Could you check a few things on this model? Use its own coordinates, in mm. A direction names the side the tool comes from. Round coordinates to 2 decimals unless told otherwise and drop trailing zeros. Write each loop counter-clockwise with the first axis right and the second up, starting at its lowest first coordinate (ties: lowest second). Pieces come first, ordered by that corner, then holes. Notation, with made-up numbers: (36, 26) - (76, 26) arc R24 ccw to (76, 61) - close; hole circle Ø8 at (16.25, -10.75). An arc over 180 degrees is marked (long way). Put each result on its own line as item: value.
Autodesk Inventor part; units mm, degrees
ref_plane "YZ Plane" through (0, 0, 0) normal (1, 0, 0) x (0, 1, 0)
ref_plane "XZ Plane" through (0, 0, 0) normal (0, 1, 0) x (-1, 0, 0)
ref_plane "XY Plane" through (0, 0, 0) normal (0, 0, 1) x (1, 0, 0)
sketch "スケッチ1" plane through (0, 0, 0) normal (0, 0, 1) x (1, 0, 0)
  circle A0 centre (0, 0) radius 27.25
  line L0 (17.5, 17.5) -> (-17.5, 17.5)
  line L1 (-17.5, 17.5) -> (-17.5, -17.5)
  line L2 (-17.5, -17.5) -> (17.5, -17.5)
  line L3 (17.5, -17.5) -> (17.5, 17.5)
  line L4 (17.5, 17.5) -> (-17.5, -17.5) construction
  line L5 (-17.5, 17.5) -> (17.5, -17.5) construction
  line L6 (1, 17.5) -> (-1, 17.5)
  line L7 (-1, 17.5) -> (-1, -17.5)
  line L8 (-1, -17.5) -> (1, -17.5)
  line L9 (1, -17.5) -> (1, 17.5)
  line L10 (1, 17.5) -> (-1, -17.5) construction
  line L11 (-1, 17.5) -> (1, -17.5) construction
  point P0 (1, -17.5)
  point P1 (1, 17.5)
  point P2 (-1, 17.5)
  point P3 (-1, -17.5)
  dimension "d0" = 54.5
  dimension "d6" = 35
  dimension "d107" = 2
  dimension "d108" = 35
extrude "押し出し1" add sketch "スケッチ1" against normal blind 3 contours A0 | L9 L2 L7 L0
sketch "スケッチ2" plane through (0, 0, 0) normal (0, 0, 1) x (1, 0, 0)
  line L0 (0, 42.4511) -> (0, -37.5489)
  line L1 (38.0038, 0) -> (-41.9962, 0)
  line L2 (27.25, 42.0143) -> (27.25, -37.9857)
  circle A0 centre (0, 0) radius 27.25
  line L3 (17.5, 17.5) -> (17.5, -17.5)
  line L4 (19.25, 25) -> (27.25, 25)
  line L5 (27.25, 25) -> (27.25, -25)
  line L6 (27.25, -25) -> (19.25, -25)
  line L7 (19.25, -25) -> (19.25, 25)
  line L8 (19.25, 25) -> (27.25, -25) construction
  line L9 (27.25, 25) -> (19.25, -25) construction
  point P0 (17.5, 0)
  point P1 (23.25, 0)
  point P2 (19.25, 0)
  point P3 (27.25, 0)
  dimension "d13" = 9.75
  dimension "d14" = 8
  dimension "d15" = 50
  dimension "d19" = 54.5
  dimension "d110" = 1.75
extrude "押し出し2" cut sketch "スケッチ2" against normal blind 10 contours L7 L4 L2 A0 | A0 L1 L7 picked at (20.3822, 11.481)
mirror "ミラー1" about plane through (0, 0, 0) normal (1, 0, 0) of "押し出し2"
sketch "スケッチ8" plane through (0, 0, 0) normal (0, 0, 1) x (1, 0, 0)
  circle A0 centre (0, 0) radius 22.375
  circle A1 centre (0, 0) radius 27.25
  line L0 (0, 31.1603) -> (0, -30.8706)
  point P0 (0, 0)
  point P1 (0, 22.375)
  point P2 (0, -22.375)
  dimension "d112" = 44.75
  dimension "d113" = 54.5
hole "穴5" at (0, 22.375, 0) at (0, -22.375, 0) direction (0, 0, -1) diameter 4.5 end through all
properties part number "Part3_A_Y" material "鋼、軟鋼"
(1) If we mould it in two halves opening along Y, with no side actions, what happens to faces 6 (the face through (0.3, 27.25, -1.48)), 7 (the face through (-9, 17.5, -1)), 8 (the face through (0, 0, -3))? For each: pulls with the +Y half, pulls with the -Y half, needs draft (parallel to the pull), parting line crosses it, or undercut.
Values found:
face 6: pulls with the +Y half
face 7: undercut
face 8: needs draft
(2) I'm going to push flat-ended pins straight in: pin 1 (1 mm diameter, centred on y = 11.5, z = -0.5, fed in from +X); pin 2 (2.5 mm diameter, centred on x = 0, y = -22.375, fed in from -Z); pin 3 (0.9 mm diameter, centred on y = 2.5, z = -1, fed in from -X); pin 4 (0.9 mm diameter, centred on x = 10, z = -2, fed in from +Y). Where does each tip first touch, or does it pass through?
Values found:
pin 1: stops at x = 19.25
pin 2: passes through
pin 3: stops at x = -19.25
pin 4: stops at y = 25.52
(3) Imagine slicing it at D-D, the plane x = -23.5. List the corners of the cut face in (y, z) for me.
Values found:
outline: (-13.8, -3) - (0, -3) - (0, 0) - (-13.8, 0) - close
(4) For faces 1 (the face through (-23, 0, -1)), 2 (the face through (-0.599, -27.243, -1.479)), 3 (the face through (0, 0, 0)), 4 (the face through (9, 17.5, -1)), 5 (the face through (19.25, 10, -1)), which set-ups out of +Z, -Z, +X, -X, +Y, -Y let a thin tool reach every point of the face, with its end or its side?
Values found:
face 1: +Z, -Z, -X, +Y
face 2: +Z, -Z, -Y
face 3: +Z, +X, -X, +Y, -Y
face 4: +Z, -Z
face 5: +Z, -Z, +X, +Y
(5) Imagine slicing it at A-A, the plane x = 0. List the corners of the cut face in (y, z) for me (3 decimals).
Values found:
outline: (-27.25, -3) - (-24.625, -3) - (-24.625, 0) - (-27.25, 0) - close; (-20.125, -3) - (20.125, -3) - (20.125, 0) - (-20.125, 0) - close; (24.625, -3) - (27.25, -3) - (27.25, 0) - (24.625, 0) - close
(6) Imagine slicing it at B-B, the plane y = 14. List the corners of the cut face in (x, z) for me.
Values found:
outline: (-19.25, -3) - (-17.5, -3) - (-17.5, 0) - (-19.25, 0) - close; (-1, -3) - (1, -3) - (1, 0) - (-1, 0) - close; (17.5, -3) - (19.25, -3) - (19.25, 0) - (17.5, 0) - close
(7) Please list where these lines run through material, in increasing order: probe 1 along Y at (x, z) = (0, -0.9) (3 decimals); probe 2 along X at (y, z) = (12, -2.6); probe 3 along X at (y, z) = (-7, -2.45). Write a range as from..to.
Values found:
probe 1: y = -27.25..-24.625, -20.125..20.125, 24.625..27.25
probe 2: x = -19.25..-17.5, -1..1, 17.5..19.25
probe 3: x = -26.34..-17.5, -1..1, 17.5..26.34
(8) Imagine slicing it at C-C, the plane z = -0.55. List the corners of the cut face in (x, y) for me (3 decimals), then the cut area to 3 significant figures.
Values found:
outline: (-27.25, 0) arc R27.25 ccw to (27.25, 0) - (19.25, 0) - (19.25, 19.287) arc R27.25 ccw to (-19.25, 19.287) - (-19.25, 0) - close; hole (-17.5, -17.5) - (-1, -17.5) - (-1, 17.5) - (-17.5, 17.5) - close; hole circle Ø4.5 at (0, -22.375); hole circle Ø4.5 at (0, 22.375); hole (1, -17.5) - (17.5, -17.5) - (17.5, 17.5) - (1, 17.5) - close
area: 933 mm^2
